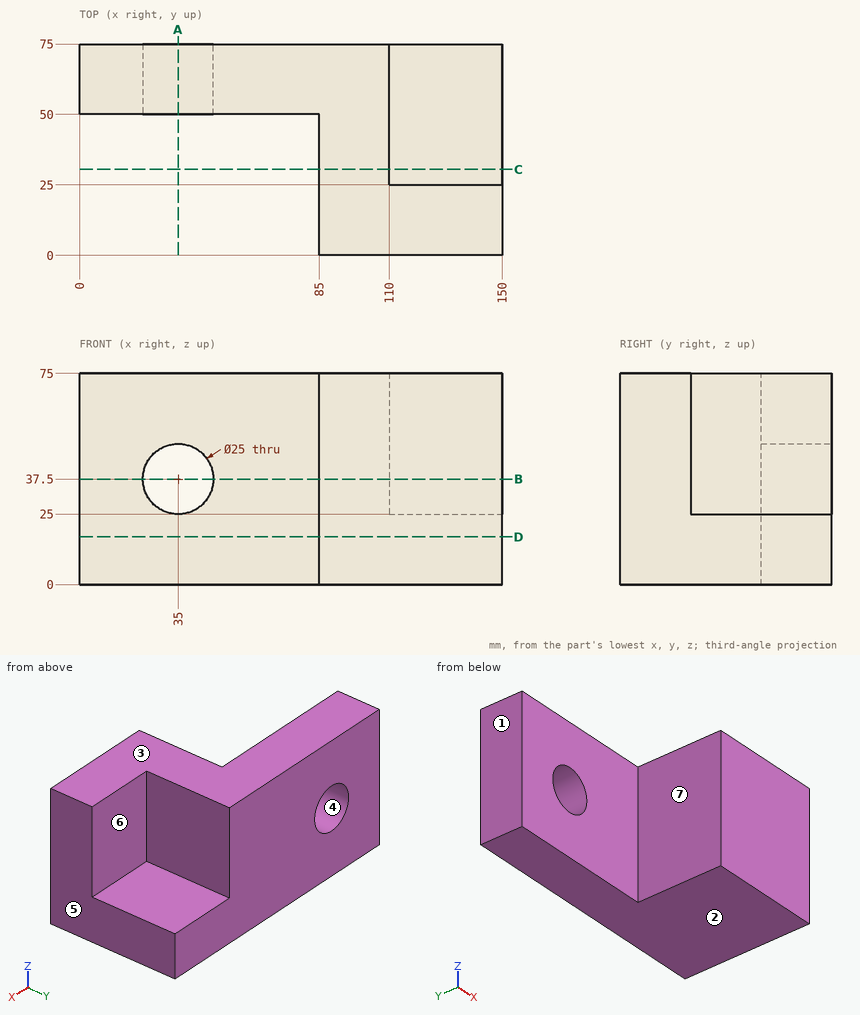
The figure shows three views and two pictorial views of one solid part (mm, origin at its lowest corner). Answer the questions. A direction names the side the tool comes from. Round coordinates to 2 decimals unless told otherwise and drop trailing zeros. Order: outer loops, then holes, each group sorted by start corner. A loop starts at its lowest first (then second) coordinate and runs counter-clockwise, first axis right, second up. Notation, with made-up numbers: M -5,-18.5 L 32,-18.5 A6 ccw 32,-11.5 Z; hole C -10.5,64.5 d10. An arc over 180 degrees is marked long. Answer in a Markdown table with one row per item. Add a question column.
1) Which of the six approach directions +Z, -Z, +X, -X, +Y, -Y give full straight-line access (tool end or side, diameter ignored) to the marked faces 5, 6 and 7?
2) Flat-ended cylindrical pins translate along their axes: pin 1 Ø12 at (x, z) = (139.5, 44.5) entering from +Y; pin 2 Ø20 at (x, y) = (120.5, 58.5) entering from +Z; pin 3 Ø6 at (y, z) = (22.5, 45) entering from -X. Find the tip coordinate at first contact, or state that the pin passes through.
3) Consider line 1 along Z through (x, y) = (35, 65); line 2 along Y through (x, z) = (49.5, 67); line 3 along X through (y, z) = (18, 7.5). Determine where each line is inside the solid, lowest interval first. Write a range as from..to.
4) The part is cut by section C-C on y = 30.5. Determine the outline of the cut face in (x, z).
5) Determine the mould class of the marked faces 1, 2, 3 and 4 for opening direction Z: pulls with the +Z half, pulls with the -Z half, needs draft (parallel to the pull), parting line crosses it, or undercut.
6) The part is cut by section A-A on x = 35. Determine the outline of the cut face in (y, z).
7) The part is cut by section D-D on z = 17. Determine the outline of the cut face in (x, y).
8) The part is cut by section B-B on z = 37.5. Determine the outline of the cut face in (x, y).
Findings below:
| question | item | result |
|---|---|---|
| 1 | face 5 | +Z, -Z, +X, +Y, -Y |
| 1 | face 6 | +Z, +X, +Y |
| 1 | face 7 | +Z, -Z, -X, -Y |
| 2 | pin 1 | stops at y = 25 |
| 2 | pin 2 | stops at z = 25 |
| 2 | pin 3 | stops at x = 85 |
| 3 | line 1 | z = 0..25, 50..75 |
| 3 | line 2 | y = 50..75 |
| 3 | line 3 | x = 85..150 |
| 4 | outline | M 85,0 L 150,0 L 150,25 L 110,25 L 110,75 L 85,75 Z |
| 5 | face 1 | needs draft |
| 5 | face 2 | pulls with the -Z half |
| 5 | face 3 | pulls with the +Z half |
| 5 | face 4 | undercut |
| 6 | outline | M 50,0 L 75,0 L 75,25 L 50,25 Z; M 50,50 L 75,50 L 75,75 L 50,75 Z |
| 7 | outline | M 0,50 L 85,50 L 85,0 L 150,0 L 150,75 L 0,75 Z |
| 8 | outline | M 0,50 L 22.5,50 L 22.5,75 L 0,75 Z; M 47.5,50 L 85,50 L 85,0 L 150,0 L 150,25 L 110,25 L 110,75 L 47.5,75 Z |
